The listing builds one solid part. Answer for the finished solid, in the listing's coordinates (mm). Face numbers are marked on the shaded views. Coordinates: 2 decimals unless noted, no trailing zeros. Order: outer loops, then holes, each group sorted by start corner. A loop starts at its lowest first (then second) coordinate and runs counter-clockwise, first axis right, second up. Notation, with made-up numbers: (48, -10) -> (65, -10) arc R34 ccw to (65, 29) -> close; hole circle Ø8 at (2, -32). An arc over 180 degrees is marked (long way). Answer in a Markdown table with one row per item.
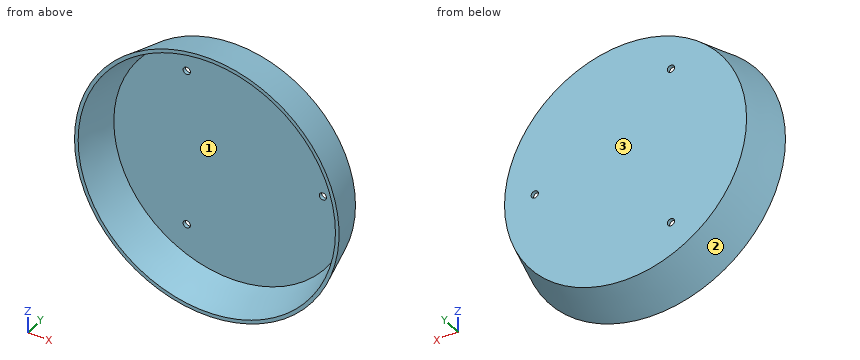
```python
from build123d import *

# Parameters (mm, degrees)
SKETCH001_R = 1.5
HOLE_DEPTH  = 25


with BuildPart() as part:
    # Sketch → Revolution (revolve)
    with BuildSketch(Plane.XY):
        Polygon((-54.6463, 0), (-53.1463, 0), (-48.887192, 16.5), (0, 16.5), (0, 18), (-50, 18), align=None)
    revolve(axis=Axis((0, 0, 0), (0, 1, 0)))

    # Sketch001 (on Face4 of Revolution) → Hole (cut)
    with BuildSketch(Plane(origin=(0, 18, 0), x_dir=(-1, 0, 0), z_dir=(0, 1, 0))):
        with Locations((-37.5, 0)):
            Circle(SKETCH001_R)
        with Locations((18.75, 32.475953)):
            Circle(SKETCH001_R)
        with Locations((18.75, -32.475953)):
            Circle(SKETCH001_R)
    extrude(amount=-HOLE_DEPTH, mode=Mode.SUBTRACT)


solid = part.part
```
(1) For a pull along X with two mould halves and no side action, classify the marked faces 1, 2 and 3 as released by +X, released by -X, zero draft, split by the parting line, or undercut.
Check values:
| item | result |
|---|---|
| face 1 | undercut |
| face 2 | split by the parting line |
| face 3 | zero draft |
(2) Find the intervals of material crossed by line 1 along Z through (x, y) = (-18.75, 17); line 2 along Z through (x, y) = (-18.75, 17.4); line 3 along Y through (x, z) = (8, -46), in increasing order. Write a range as from..to.
Check values:
| item | result |
|---|---|
| line 1 | -46.63..-33.98, -30.98..30.98, 33.98..46.63 |
| line 2 | -46.52..-33.98, -30.98..30.98, 33.98..46.52 |
| line 3 | 16.5..18 |
(3) Flat-ended cylindrical pins translate along their axes: pin 1 (5 mm diameter, centred on x = -22, y = 13, fed in from +Z); pin 2 (8 mm diameter, centred on x = -43, y = 13, fed in from -Z) (3 decimals); pin 3 (1 mm diameter, centred on y = 14.5, z = 38, fed in from -X) (3 decimals). Find the tip coordinate at first contact, or state that the pin passes through.
Check values:
| item | result |
|---|---|
| pin 1 | z = 47.65 |
| pin 2 | z = -33.575 |
| pin 3 | x = -34.455 |
(4) A cutting plane is placed at C-C, the plane y = 14.75. Determine the outline of the cut face in (x, z), then the cut area to 3 significant figures.
Check values:
| item | result |
|---|---|
| outline | circle Ø101.68 at (0, 0); hole circle Ø98.68 at (0, 0) |
| area | 472 mm² |
(5) A cutting plane is placed at B-B, the plane x = 0. Determine the outline of the cut face in (y, z), then the cut area to 3 significant figures.
Check values:
| item | result |
|---|---|
| outline | (0, -54.65) -> (18, -50) -> (18, 50) -> (0, 54.65) -> (0, 53.15) -> (16.5, 48.89) -> (16.5, -48.89) -> (0, -53.15) -> close |
| area | 200 mm² |
(6) A cutting plane is placed at A-A, the plane z = 0. Determine the outline of the cut face in (x, y), then the cut area to 3 significant figures.
Check values:
| item | result |
|---|---|
| outline | (-54.65, 0) -> (-53.15, 0) -> (-48.89, 16.5) -> (36, 16.5) -> (36, 18) -> (-50, 18) -> close; (39, 16.5) -> (48.89, 16.5) -> (53.15, 0) -> (54.65, 0) -> (50, 18) -> (39, 18) -> close |
| area | 196 mm² |
(7) A cutting plane is placed at D-D, the plane x = -18.75. Count the separate pieces of the cut face and the enclosed holes in it, then the cut area to 3 significant figures.
Check values:
| item | result |
|---|---|
| separate pieces | 3 |
| enclosed holes | 0 |
| area | 184 mm² |
